Could you check a few things on this model? Use its own coordinates, in mm. Face numbers are marked on the shaded views. A direction names the side the tool comes from. Round coordinates to 2 decimals unless told otherwise and drop trailing zeros. Order: outer loops, then holes, each group sorted by start corner. A loop starts at its lowest first (then second) coordinate and runs counter-clockwise, first axis right, second up. Notation, with made-up numbers: M 58,21 L 87,21 A17 ccw 87,47 Z; hole C -26,32 d4. An arc over 180 degrees is marked long. Write each question's results on one line, items separated by ' | '. Start each with the question number.
1. Suppose I cut it at C-C on y = 10.5. Write out the boundary of the cut face in (x, z).
2. I'm going to push flat-ended pins straight in: pin 1 (14.5 mm diameter, centred on y = 24.5, z = 11.5, fed in from +X); pin 2 (20.5 mm diameter, centred on x = 22.5, z = 42, fed in from +Y); pin 3 (6 mm diameter, centred on y = -7, z = 62, fed in from -X); pin 4 (24.5 mm diameter, centred on x = 16, z = 89.5, fed in from -Y). Where does each tip first touch, or does it pass through?
3. Suppose I cut it at B-B on x = 70. Write out the boundary of the cut face in (y, z), and give its area (3 significant figures).
4. For the marked faces 1, 2, 3, 4 and 5, which set-ups out of +Z, -Z, +X, -X, +Y, -Y let a thin tool reach every point of the face, with its end or its side?
5. Please list where these lines run through material, in increasing order: L1, parallel to X at y = 24.5, z = 93; L2, parallel to Y at x = 23, z = 69.5; L3, parallel to Z at x = 24, y = -24.
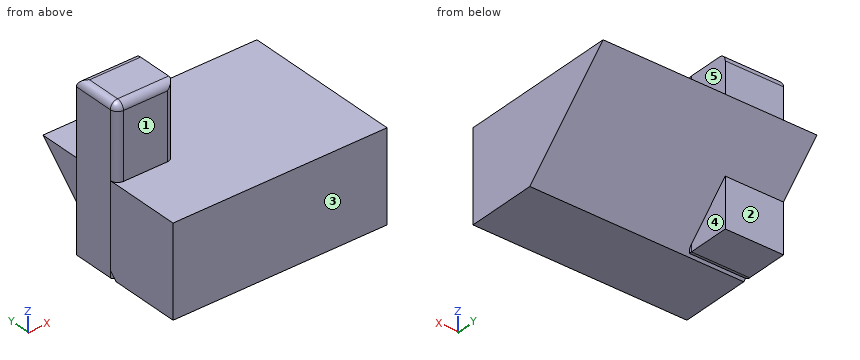
from build123d import *

# Parameters (mm, degrees)
F0_W     = 40.850177
F0_H     = 34.370493
F1_DEPTH = 114.554
F2_R     = 5.08
F4_DEPTH = 150


with BuildPart() as f1:
    # F0 (on Top) → F1 (new body)
    with BuildSketch(Plane.XY):
        with Locations((20.425088, 17.185246)):
            Rectangle(F0_W, F0_H)
    extrude(amount=F1_DEPTH)

    # F2
    f2_edges = [f1.edges().sort_by_distance(p)[0] for p in [
        (20.425089, 0, 114.554),
        (20.425089, 34.370493, 114.554),
        (0, 0, 57.277),
        (0, 17.185247, 114.554),
        (40.850177, 0, 57.277),
        (20.425089, 0, 0),
    ]]
    fillet(f2_edges, radius=F2_R)

    # F3 (on Right) → F4 (join)
    with BuildSketch(Plane.YZ):
        Polygon((-49.08682, 0), (0, 0), (63.275978, 63.303202), (-49.08682, 63.303202), align=None)
    extrude(amount=F4_DEPTH)


solid = f1.part
Filled sheet:
1) outline: M 0,0 L 40.85,0 L 40.85,10.5 L 150,10.5 L 150,63.3 L 40.85,63.3 L 40.85,114.55 L 5.08,114.55 A5.08 ccw 0,109.47 Z
2) pin 1: stops at x = 40.85 | pin 2: stops at y = 52.23 | pin 3: stops at x = 0 | pin 4: stops at y = 0
3) outline: M -49.09,0 L 0,0 L 63.28,63.3 L -49.09,63.3 Z | area: 5,110 mm^2
4) face 1: +Z, +X, -X, -Y | face 2: -Z, +X, -X, +Y | face 3: +Z, -Z, +X, -X, -Y | face 4: -Z, +X, +Y | face 5: +Z, +X, +Y, -Y
5) L1: x = 0 to 40.85 | L2: y = 0 to 34.37 | L3: z = 0 to 63.3
